Input: part model. Units: mm. Frame: model coordinates. Face numbers are marked on the shaded views. A direction names the side the tool comes from. Round coordinates to 2 decimals unless told otherwise and drop trailing zeros. Write each loop counter-clockwise with the first axis right and the second up, starting at its lowest first coordinate (ties: lowest second). Pieces come first, ordered by that corner, then holes. Notation, with made-up numbers: (71.5, -36.5) -> (98.5, -36.5) arc R13 cw to (98.5, -25.5) -> close; hole circle Ø6 at (25, 54). An arc over 180 degrees is marked (long way). Write item = value, one per line. Start each with the question number.
Autodesk Inventor part; units mm, degrees
ref_plane "Start Plane" through (0, 0, -10) normal (0, 0, 1) x (1, 0, 0)
ref_plane "End Plane" through (0, 0, 66.3002) normal (0, 0, 1) x (1, 0, 0)
ref_plane "Work Plane4" through (7, 153.7024, 115.5399) normal (0, -0.3241, 0.946) x (1, 0, 0)
ref_plane "Start Plane" through (0, 0, -10) normal (0, 0, 1) x (1, 0, 0)
ref_plane "End Plane" through (0, 0, 66.3002) normal (0, 0, 1) x (1, 0, 0)
sketch "Sketch" plane through (0, 0, 0) normal (0, 0, 1) x (1, 0, 0)
  line L0 (-10, -7) -> (-10, 7)
  line L1 (-7, 10) -> (7, 10)
  line L2 (10, 7) -> (10, -7)
  line L3 (7, -10) -> (-7, -10)
  arc A0 (-10, -7) -> (-7, -10) centre (-7, -7) ccw
  arc A1 (-7, 10) -> (-10, 7) centre (-7, 7) ccw
  arc A2 (10, 7) -> (7, 10) centre (7, 7) ccw
  arc A3 (7, -10) -> (10, -7) centre (7, -7) ccw
  arc A4 (-7, 8) -> (-8, 7) centre (-7, 7) ccw
  line L4 (-7, 8) -> (7, 8)
  arc A5 (8, 7) -> (7, 8) centre (7, 7) ccw
  line L5 (8, 7) -> (8, -7)
  arc A6 (7, -8) -> (8, -7) centre (7, -7) ccw
  line L6 (7, -8) -> (-7, -8)
  arc A7 (-8, -7) -> (-7, -8) centre (-7, -7) ccw
  line L7 (-8, -7) -> (-8, 7)
  line L8 (0, 14.8698) -> (0, -14.8698) construction
  line L9 (-14.8698, 0) -> (14.8698, 0) construction
  dimension "d7" = 3
  dimension "d10" = 20
  dimension "d11" = 20
  dimension "d12" = 2
  dimension "d15" = 10
  dimension "d16" = 10
extrude "Body" add sketch "Sketch" along normal up to surface (76.3002 mm away) from surface at -10
sketch "Sketch3" plane through (0, 0, 0) normal (0, 0, 1) x (1, 0, 0)
  line L0 (0, 0) -> (10, 0)
ref_plane "Work Plane3" through (0, 0, 0) normal (0, -1, 0) x (1, 0, 0)
sketch "Sketch4" plane through (0, 0, 0) normal (0, -1, 0) x (1, 0, 0)
  line L0 (-2, -10) -> (12, -10)
  line L1 (-2, 66.3002) -> (12, 66.3002)
  dimension "d18" = 76.3002
ref_plane "Work Plane4" through (7, 153.7024, 115.5399) normal (0, -0.3241, 0.946) x (1, 0, 0)
split "Split1" plane through (7, 153.7024, 115.5399) removes the side toward (0, -0.3241, 0.946)
ref_plane "Work Plane6" through (0, 10, -10) normal (0, -0.7071, -0.7071) x (1, 0, 0)
split "Split3" plane through (0, 10, -10) removes the side toward (0, -0.7071, -0.7071)
sketch "Sketch6" plane through (10, 7, 65.2722) normal (1, 0, 0) x (0, 0, -1)
  point P0 (65.2722, -10.933)
hole "Hole2" at (10, -3.933, 0) direction (-1, 0, 0) diameter 6.6 depth 2
sketch "Sketch7" plane through (-8, 7, 65.2722) normal (1, 0, 0) x (0, 0, -1)
  point P0 (65.2722, -10.933)
hole "Hole3" at (-8, -3.933, 0) direction (-1, 0, 0) diameter 6.6 end through all
equation "\"d7\" = G_IR"
equation "\"d10\" = G_H"
equation "\"d11\" = G_W"
equation "\"d12\" = G_T"
equation "\"d15\" = 0.5 * d10"
equation "\"d16\" = 0.5 * d11"
equation "\"d3\" = G_L"
equation "\"G_W\" = 20"
equation "\"G_H\" = 20"
equation "\"G_T\" = 2"
equation "\"G_IR\" = 3"
equation "\"G_L\" = d18"
equation "\"G_OFFSET_END\" = -7.14425"
equation "\"d14\" = G_OFFSET_END + B_L"
equation "\"B_L\" = 73.44444"
properties part number "ISO 12633-2 - 20x20x2 - 76,3" material "Steel, Mild"
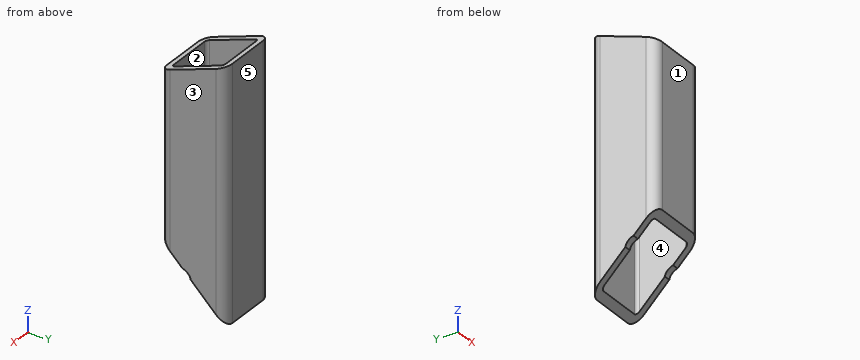
1. Section C-C (y = -5). Output: boundary loops of the cut face in (x, z), then the cut area to 3 significant figures.
2. Mould query, pull axis X, two halves, no side actions, for the marked faces 3, 4 and 5. Classes: pulls with the +X half, pulls with the -X half, needs draft (parallel to the pull), parting line crosses it, or undercut.
3. Reachability of the marked faces 1 and 2 from +Z, -Z, +X, -X, +Y, -Y: full face, straight path, thin tool, end or side. Return the list, or none.
4. Section D-D (y = 3). Output: boundary loops of the cut face in (x, z).
5. Pin query (flat end, axial travel): P1, Ø1, axis at x = 7, y = 2, coming from the -Z side; P2, Ø12, axis at x = 2, y = 3, coming from the -Z side. Return the tip coordinate at first contact, or that it passes through.
6. Line query: line 1 along X through (y, z) = (5.25, 12); line 2 along Y through (x, z) = (2.5, -7). Output: solid intervals per line, ascending.
7. Section A-A (z = 13). Output: boundary loops of the cut face in (x, y), then the cut area to 3 significant figures.
Check sheet entries:
q1.outline = (-10, 5) -> (-8, 5) -> (-8, 61.17) -> (-10, 61.17) -> close; (8, 5) -> (10, 5) -> (10, 61.17) -> (8, 61.17) -> close
q1.area = 225 mm2
q2.face_3 = pulls with the +X half
q2.face_4 = undercut
q2.face_5 = needs draft
q3.face_1 = +Z, -Z, +X, -X, -Y
q3.face_2 = +Z, -Z
q4.outline = (-10, -3) -> (-8, -3) -> (-8, 63.91) -> (-10, 63.91) -> close; (8, -3) -> (10, -3) -> (10, 63.91) -> (8, 63.91) -> close
q5.P1 = through
q5.P2 = -9
q6.line_1 = -10 to -8, 8 to 10
q6.line_2 = 8 to 10
q7.outline = (-10, -7) arc R3 ccw to (-7, -10) -> (7, -10) arc R3 ccw to (10, -7) -> (10, 7) arc R3 ccw to (7, 10) -> (-7, 10) arc R3 ccw to (-10, 7) -> close; hole (-8, -7) arc R1 ccw to (-7, -8) -> (7, -8) arc R1 ccw to (8, -7) -> (8, 7) arc R1 ccw to (7, 8) -> (-7, 8) arc R1 ccw to (-8, 7) -> close
q7.area = 137 mm2
